Autodesk Inventor part; units mm, degrees
ref_plane "YZ Plane" through (0, 0, 0) normal (1, 0, 0) x (0, 1, 0)
ref_plane "XZ Plane" through (0, 0, 0) normal (0, 1, 0) x (-1, 0, 0)
ref_plane "XY Plane" through (0, 0, 0) normal (0, 0, 1) x (1, 0, 0)
sketch "Sketch1" plane through (0, 0, 0) normal (0, 0, 1) x (1, 0, 0)
  line L0 (-254.2423, -28) -> (254.2423, -28)
  line L1 (282.2423, 0) -> (282.2423, 28)
  line L2 (282.2423, 28) -> (-254.2423, 28) construction
  line L3 (-282.2423, 0) -> (-282.2423, 0)
  line L4 (-282.2423, -28) -> (282.2423, 28) construction
  line L5 (282.2423, -28) -> (-282.2423, 28) construction
  arc A0 (-254.2423, 28) -> (-282.2423, 0) centre (-254.2423, 0) ccw
  arc A1 (-282.2423, 0) -> (-254.2423, -28) centre (-254.2423, 0) ccw
  circle A2 centre (-134.2423, 0) radius 7
  circle A3 centre (-149.7986, 15.5563) radius 2.1
  line L6 (-134.2423, 0) -> (-149.7986, 15.5563) construction
  line L7 (-134.2423, 0) -> (-254.2423, 0) construction
  circle A4 centre (-149.7986, -15.5563) radius 2.1
  circle A5 centre (-118.6859, -15.5563) radius 2.1
  circle A6 centre (-118.6859, 15.5563) radius 2.1
  arc A7 (254.2423, -28) -> (282.2423, 0) centre (254.2423, 0) ccw
  circle A8 centre (254.2423, 0) radius 7
  line L8 (282.2423, 28) -> (282.2423, 92)
  line L9 (282.2423, 92) -> (226.2423, 92)
  line L10 (226.2423, 92) -> (226.2423, 28)
  line L11 (226.2423, 28) -> (-254.2423, 28)
  circle A9 centre (254.2423, 56) radius 19.5
  circle A10 centre (-254.2423, 0) radius 7
  circle A11 centre (-263.1865, 8) radius 2
  circle A12 centre (-266.2237, -0.6677) radius 2
  circle A13 centre (-262.2423, -8.9443) radius 2
  circle A14 centre (-253.5746, -11.9814) radius 2
  circle A15 centre (-245.298, -8) radius 2
  circle A16 centre (-242.2609, 0.6677) radius 2
  circle A17 centre (-246.2423, 8.9443) radius 2
  circle A18 centre (-254.91, 11.9814) radius 2
  line L12 (-134.2423, 0) -> (254.2423, 56) construction
  point P0 (0, 0)
  point P1 (-282.2423, 0)
  dimension "d1" = 56
  dimension "d3" = 28
  dimension "d4" = 14
  dimension "d5" = 120
  dimension "d6" = 4.2
  dimension "d7" = 45
  dimension "d8" = 22
  dimension "d11" = 360
  dimension "d13" = 28
  dimension "d16" = 14
  dimension "d17" = 64
  dimension "d18" = 56
  dimension "d19" = 39
  dimension "d20" = 56
  dimension "d21" = 14
  dimension "d22" = 4
  dimension "d24" = 8
  dimension "d27" = 360
  dimension "d50" = 12
  dimension "d65" = 392.5
extrude "Extrusion1" add sketch "Sketch1" along normal blind 3
sketch "Sketch2" plane through (0, 0, 3) normal (0, 0, 1) x (1, 0, 0)
  line L0 (226.2423, 28) -> (-254.2423, 28) construction
  circle A0 centre (-254.2423, 24) radius 2
  circle A1 centre (-230.2423, 24) radius 2
  circle A2 centre (-206.2423, 24) radius 2
  circle A3 centre (-182.2423, 24) radius 2
  circle A4 centre (-158.2423, 24) radius 2
  circle A5 centre (-134.2423, 24) radius 2
  circle A6 centre (-110.2423, 24) radius 2
  circle A7 centre (-86.2423, 24) radius 2
  circle A8 centre (-62.2423, 24) radius 2
  circle A9 centre (-38.2423, 24) radius 2
  circle A10 centre (-14.2423, 24) radius 2
  line L1 (0, 28) -> (0, -28) construction
  line L2 (-254.2423, -28) -> (254.2423, -28) construction
  circle A11 centre (254.2423, 24) radius 2
  circle A12 centre (230.2423, 24) radius 2
  circle A13 centre (206.2423, 24) radius 2
  circle A14 centre (182.2423, 24) radius 2
  circle A15 centre (158.2423, 24) radius 2
  circle A16 centre (134.2423, 24) radius 2
  circle A17 centre (110.2423, 24) radius 2
  circle A18 centre (86.2423, 24) radius 2
  circle A19 centre (62.2423, 24) radius 2
  circle A20 centre (38.2423, 24) radius 2
  circle A21 centre (14.2423, 24) radius 2
  arc A22 (-254.2423, 28) -> (-254.2423, -28) centre (-254.2423, 0) ccw construction
  arc A23 (254.2423, -28) -> (282.2423, 0) centre (254.2423, 0) ccw construction
  line L3 (-282.2423, 0) -> (282.2423, 0) construction
  line L4 (226.2423, -28) -> (-254.2423, -28) construction
  circle A24 centre (-254.2423, -24) radius 2
  circle A25 centre (-230.2423, -24) radius 2
  circle A26 centre (-206.2423, -24) radius 2
  circle A27 centre (-182.2423, -24) radius 2
  circle A28 centre (-158.2423, -24) radius 2
  circle A29 centre (-134.2423, -24) radius 2
  circle A30 centre (-110.2423, -24) radius 2
  circle A31 centre (-86.2423, -24) radius 2
  circle A32 centre (-62.2423, -24) radius 2
  circle A33 centre (-38.2423, -24) radius 2
  circle A34 centre (-14.2423, -24) radius 2
  circle A35 centre (62.2423, -24) radius 2
  circle A36 centre (38.2423, -24) radius 2
  circle A37 centre (14.2423, -24) radius 2
  circle A38 centre (86.2423, -24) radius 2
  circle A39 centre (110.2423, -24) radius 2
  circle A40 centre (134.2423, -24) radius 2
  circle A41 centre (158.2423, -24) radius 2
  circle A42 centre (182.2423, -24) radius 2
  circle A43 centre (206.2423, -24) radius 2
  circle A44 centre (230.2423, -24) radius 2
  circle A45 centre (254.2423, -24) radius 2
  circle A46 centre (230.2423, 88) radius 2.1
  line L5 (226.2423, 92) -> (226.2423, 28) construction
  line L6 (282.2423, 92) -> (226.2423, 92) construction
  circle A47 centre (278.2423, 88) radius 2.1
  line L7 (282.2423, 0) -> (282.2423, 92) construction
  circle A48 centre (278.2423, 24) radius 2.1
  point P0 (0, 0)
  point P1 (254.2423, 28)
  dimension "d29" = 4
  dimension "d30" = 4
  dimension "d33" = 24
  dimension "d38" = 4.2
  dimension "d39" = 4
  dimension "d40" = 4
  dimension "d41" = 4.2
  dimension "d42" = 4
  dimension "d43" = 4
  dimension "d56" = 4.2
extrude "Extrusion2" cut sketch "Sketch2" against normal through all
sketch "Sketch3" plane through (0, 0, 3) normal (0, 0, 1) x (1, 0, 0)
  circle A0 centre (-134.2423, 0) radius 7 construction
  circle A1 centre (-90.2423, 17) radius 2.1
  line L0 (-134.2423, 0) -> (-127.2423, 0) construction
  circle A2 centre (-134.2423, 0) radius 7 construction
  line L1 (-134.2423, 0) -> (-134.2423, 7) construction
  circle A3 centre (-90.2423, -17) radius 2.1
  circle A4 centre (-178.2423, 17) radius 2.1
  circle A5 centre (-178.2423, -17) radius 2.1
  point P0 (0, 0)
  dimension "d51" = 4.2
  dimension "d52" = 44
  dimension "d53" = 17
extrude "Extrusion3" cut sketch "Sketch3" against normal through all
fillet "Fillet1" radius 4 2 edges at (226.2423, 92, 1.5) (282.2423, 92, 1.5)
sketch "Sketch4" plane through (0, 0, 3) normal (0, 0, 1) x (1, 0, 0)
  circle A0 centre (-149.7986, 15.5563) radius 2.1
  circle A1 centre (-118.6859, 15.5563) radius 2.1
  circle A2 centre (-118.6859, -15.5563) radius 2.1
  circle A3 centre (-149.7986, -15.5563) radius 2.1
  point P0 (0, 0)
hole "Hole1" at (-149.7986, 15.5563, 3) at (-149.7986, -15.5563, 3) at (-118.6859, -15.5563, 3) at (-118.6859, 15.5563, 3) direction (0, 0, -1) diameter 4.2 end through all countersink diameter 8 countersink angle 90
sketch "Sketch5" plane through (0, 0, 0) normal (0, 0, -1) x (-1, 0, 0)
  circle A0 centre (178.2423, -17) radius 2.1
  circle A1 centre (90.2423, -17) radius 2.1
  circle A2 centre (90.2423, 17) radius 2.1
  circle A3 centre (178.2423, 17) radius 2.1
  circle A4 centre (158.2423, 24) radius 2
  circle A5 centre (62.2423, 24) radius 2
  circle A6 centre (62.2423, -24) radius 2
  circle A7 centre (110.2423, -24) radius 2
  circle A8 centre (206.2423, 24) radius 2
  circle A9 centre (230.2423, -24) radius 2
  circle A10 centre (-38.2423, -24) radius 2
  circle A11 centre (-62.2423, -24) radius 2
  circle A12 centre (-110.2423, 24) radius 2
  circle A13 centre (-206.2423, 24) radius 2
  circle A14 centre (-254.2423, -24) radius 2
  circle A15 centre (-86.2423, -24) radius 2
  circle A16 centre (-254.2423, 24) radius 2
  circle A17 centre (-278.2423, 88) radius 2.1
  circle A18 centre (-134.2423, 24) radius 2
  circle A19 centre (-158.2423, -24) radius 2
  circle A20 centre (-134.2423, -24) radius 2
  circle A21 centre (-206.2423, -24) radius 2
  circle A22 centre (182.2423, -24) radius 2
  circle A23 centre (134.2423, -24) radius 2
  circle A24 centre (38.2423, -24) radius 2
  circle A25 centre (38.2423, 24) radius 2
  circle A26 centre (134.2423, 24) radius 2
  circle A27 centre (182.2423, 24) radius 2
  circle A28 centre (86.2423, 24) radius 2
  circle A29 centre (230.2423, 24) radius 2
  circle A30 centre (86.2423, -24) radius 2
  circle A31 centre (158.2423, -24) radius 2
  circle A32 centre (206.2423, -24) radius 2
  circle A33 centre (-182.2423, -24) radius 2
  circle A34 centre (-62.2423, 24) radius 2
  circle A35 centre (-86.2423, 24) radius 2
  circle A36 centre (-182.2423, 24) radius 2
  circle A37 centre (-38.2423, 24) radius 2
  circle A38 centre (-14.2423, 24) radius 2
  circle A39 centre (-14.2423, -24) radius 2
  circle A40 centre (-230.2423, 24) radius 2
  circle A41 centre (-158.2423, 24) radius 2
  circle A42 centre (-230.2423, 88) radius 2.1
  circle A43 centre (-110.2423, -24) radius 2
  circle A44 centre (-230.2423, -24) radius 2
  circle A45 centre (254.2423, -24) radius 2
  circle A46 centre (254.2423, 24) radius 2
  circle A47 centre (14.2423, -24) radius 2
  circle A48 centre (14.2423, 24) radius 2
  circle A49 centre (110.2423, 24) radius 2
  circle A50 centre (-278.2423, 24) radius 2.1
  arc A51 (-278.2423, 92) -> (-282.2423, 88) centre (-278.2423, 88) ccw
  line L0 (-282.2423, 0) -> (-282.2423, 88)
  arc A52 (-282.2423, 0) -> (-254.2423, -28) centre (-254.2423, 0) ccw
  line L1 (254.2423, -28) -> (-254.2423, -28)
  arc A53 (254.2423, -28) -> (254.2423, 28) centre (254.2423, 0) ccw
  line L2 (-226.2423, 28) -> (254.2423, 28)
  line L3 (-226.2423, 88) -> (-226.2423, 28)
  arc A54 (-226.2423, 88) -> (-230.2423, 92) centre (-230.2423, 88) ccw
  line L4 (-278.2423, 92) -> (-230.2423, 92)
  circle A55 centre (134.2423, 0) radius 7
  circle A56 centre (149.7986, 15.5563) radius 2.1
  circle A57 centre (149.7986, -15.5563) radius 2.1
  circle A58 centre (118.6859, -15.5563) radius 2.1
  circle A59 centre (118.6859, 15.5563) radius 2.1
  circle A60 centre (-254.2423, 56) radius 19.5
  circle A61 centre (242.2609, 0.6677) radius 2
  circle A62 centre (254.91, 11.9814) radius 2
  circle A63 centre (246.2423, 8.9443) radius 2
  circle A64 centre (245.298, -8) radius 2
  circle A65 centre (253.5746, -11.9814) radius 2
  circle A66 centre (262.2423, -8.9443) radius 2
  circle A67 centre (266.2237, -0.6677) radius 2
  circle A68 centre (263.1865, 8) radius 2
  circle A69 centre (254.2423, 0) radius 7
  circle A70 centre (-254.2423, 0) radius 7
  point P0 (0, 0)
hole "Hole2" at (-254.2423, 24, 0) at (-254.2423, -24, 0) direction (0, 0, 1) diameter 4.12 end through all countersink diameter 8 countersink angle 90
hole "Hole3" at (230.2423, 88, 3) at (278.2423, 88, 3) direction (0, 0, -1) diameter 4.12 end through all countersink diameter 8 countersink angle 90
equation "\"d3\" = 0.5 * d1"
equation "\"d13\" = d3"
properties part number "FirstStageArmBar1" material "Aluminum 6061"
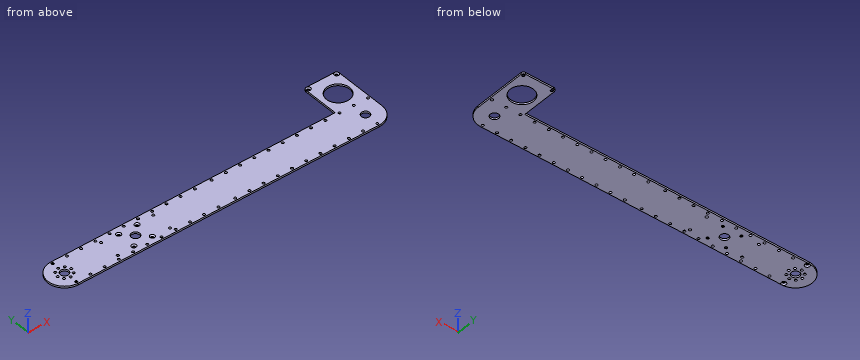
Verification items for the finished model (mm, model axes). Coordinates: 2 decimals unless noted, no trailing zeros. Order: outer loops, then holes, each group sorted by start corner. A loop starts at its lowest first (then second) coordinate and runs counter-clockwise, first axis right, second up. Notation, with made-up numbers: M 77,-18 L 102,-18 A11 cw 102,-10 Z; hole C 62,53 d5. An arc over 180 degrees is marked long. One line per item, written item: value. Start each with the question number.
Item 1: Depth check by flat-ended pin: P1, Ø2.5, axis at x = -118.69, y = 15.56, coming from the -Z side; P2, Ø5, axis at x = -149.8, y = -15.56, coming from the +Z side. Enter the tip coordinate at first touch or a pass-through.
Item 2: Sectioned sample at B-B on z = 0.55. Give the number of separate pieces and of enclosed holes in the cut face, then the cut area to 3 significant figures.
Item 3: Thickness scan on probe 1 along X at (y, z) = (2.5, 2.55); probe 2 along Y at (x, z) = (-177.5, 1); probe 3 along X at (y, z) = (2, 2). Record the ranges inside material, lowest first.
Item 4: Sectioned sample at C-C on x = -171. Record the cut outline in (y, z), then the cut area to 3 significant figures.
Item 5: Sectioned sample at A-A on y = 56. Record the cut outline in (x, z), then the cut area to 3 significant figures.
Calculated:
1. P1: through
1. P2: z = 1.5
2. separate pieces: 1
2. enclosed holes: 67
2. area: 32,200 mm^2
3. probe 1: -282.13 to -260.78, -247.7 to -243.06, -241.46 to -140.78, -127.7 to 247.7, 260.78 to 282.24
3. probe 2: -28 to -18.96, -15.04 to 15.04, 18.96 to 28
3. probe 3: -282.17 to -260.95, -247.53 to -243.75, -240.77 to -140.95, -127.53 to 247.53, 260.95 to 282.24
4. outline: M -28,0 L 28,0 L 28,3 L -28,3 Z
4. area: 168 mm^2
5. outline: M 226.24,0 L 234.74,0 L 234.74,3 L 226.24,3 Z; M 273.74,0 L 282.24,0 L 282.24,3 L 273.74,3 Z
5. area: 51.0 mm^2
